Answer from the drawing. Dimensions are ordinates in mm from the lowest x, y and z of the part. Give positions to 0.01 mm unless a question says otherwise; leave off trailing zeros. Loops run counter-clockwise (first coordinate to the right, second up) from the corner with the lowest first, then second, coordinate; pieces in that order, holes last. Notation, with made-up numbers: (62.5, 66) - (115.5, 66) arc R7 ccw to (115.5, 70) - close; hole circle Ø9 at (9.25, 49). An arc over 180 degrees is marked (long way). Write each question's results on one line, items separated by ' | '. Start each with the question number.
Q1. The part is cut by section B-B, the plane y = 13.25. Write down the section's boundary in (x, z).
Q2. Determine the mould class of the marked faces 1, 2, 3 and 4 for opening direction X: +X half, -X half, draft (parallel to the pull), parting line (faces both ways), or undercut.
Q3. Find the intervals of material crossed by line 1 (Z direction, x = 1.05, y = 21.5); line 2 (X direction, y = 15, z = 6.25); line 3 (Y direction, x = 0.25, z = 5.5), in increasing order. Write a range as from..to.
Q4. The part is cut by section A-A, the plane z = 4.25. State how many separate pieces and enclosed holes the cut face has, plus the area to 3 significant figures.
Q5. The part is cut by section D-D, the plane x = 2.5. Write down the section's boundary in (y, z).
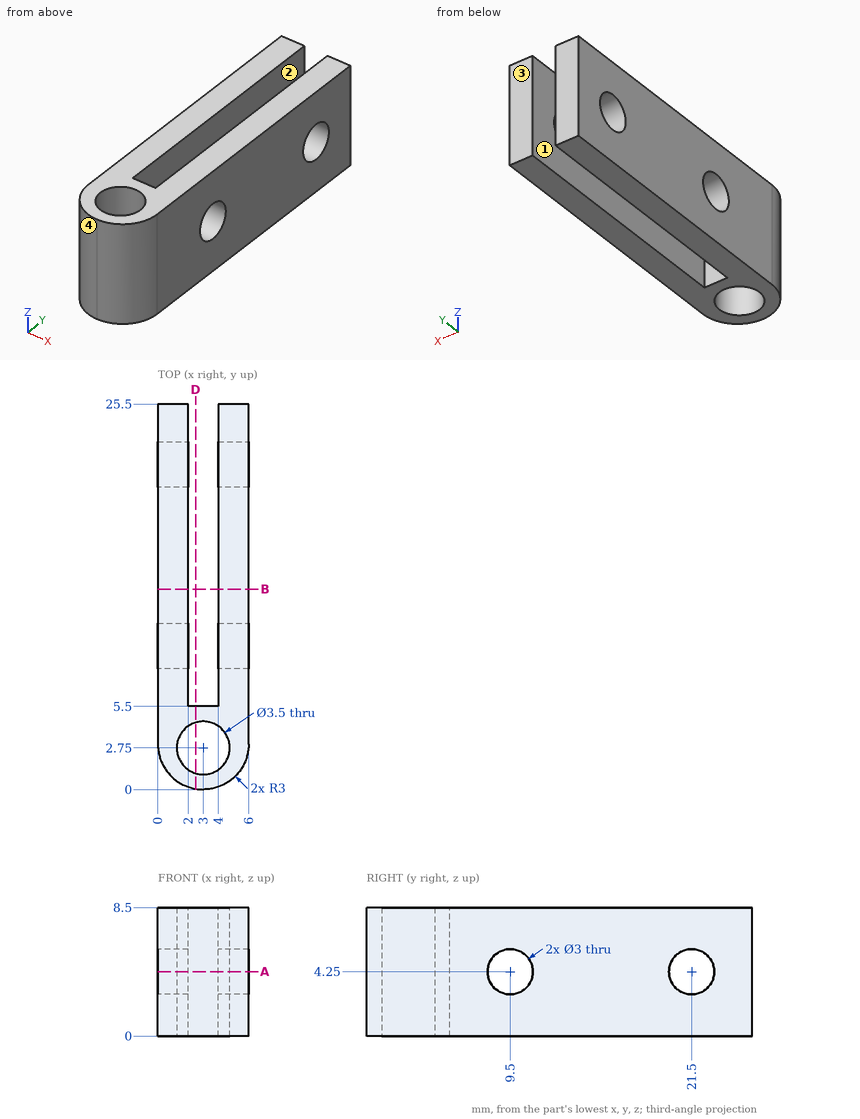
Check sheet entries:
1) outline: (0, 0) - (2, 0) - (2, 8.5) - (0, 8.5) - close; (4, 0) - (6, 0) - (6, 8.5) - (4, 8.5) - close
2) face 1: undercut | face 2: undercut | face 3: draft | face 4: -X half
3) line 1: z = 0..2.75, 5.75..8.5 | line 2: x = 0..2, 4..6 | line 3: y = 1.8..8.67, 10.33..20.67, 22.33..25.5
4) separate pieces: 5 | enclosed holes: 1 | area: 75.5 mm^2
5) outline: (0.04, 0) - (1.07, 0) - (1.07, 8.5) - (0.04, 8.5) - close; (4.43, 0) - (5.5, 0) - (5.5, 8.5) - (4.43, 8.5) - close
